from build123d import *

# Parameters (mm, degrees)
BOSS_EXTRUDE1_DEPTH   = 8
FILLET1_R             = 5
FILLET3_R             = 0.5
M4_TAPPED_HOLE1_D     = 3.3
M4_TAPPED_HOLE1_DEPTH = 14.6
M4_TAPPED_HOLE1_TIP   = 0.991420021
M4_TAPPED_HOLE2_D     = 3.3
M4_TAPPED_HOLE2_DEPTH = 14.6
M4_TAPPED_HOLE2_TIP   = 0.991420021


with BuildPart() as part:
    # Sketch1 → Boss-Extrude1 (new body)
    with BuildSketch(Plane.XY):
        Polygon((0, 0), (80, 0), (80, 10), (12, 50), (0, 50), align=None)
    extrude(amount=BOSS_EXTRUDE1_DEPTH)

    # Fillet1
    fillet1_edges = [part.edges().sort_by_distance(p)[0] for p in [
        (12, 50, 4),
        (80, 10, 4),
    ]]
    fillet(fillet1_edges, radius=FILLET1_R)

    # Fillet3
    fillet3_edges = [part.edges().sort_by_distance(p)[0] for p in [
        (0, 50, 4),
        (80, 0, 4),
        (0, 0, 4),
    ]]
    fillet(fillet3_edges, radius=FILLET3_R)

    # M4 Tapped Hole1
    with Locations(Plane.ZY):
        with Locations((4, 43.5), (4, 6)):
            Hole(M4_TAPPED_HOLE1_D / 2, depth=M4_TAPPED_HOLE1_DEPTH)
            with Locations((0, 0, -(M4_TAPPED_HOLE1_DEPTH + M4_TAPPED_HOLE1_TIP / 2))):  # 118° drill point
                Cone(0, M4_TAPPED_HOLE1_D / 2, M4_TAPPED_HOLE1_TIP, mode=Mode.SUBTRACT)

    # M4 Tapped Hole2
    with Locations(Plane(origin=(0, 0, 0), x_dir=(-1, 0, 0), z_dir=(0, -1, 0))):
        with Locations((-20, -4), (-65, -4)):
            Hole(M4_TAPPED_HOLE2_D / 2, depth=M4_TAPPED_HOLE2_DEPTH)
            with Locations((0, 0, -(M4_TAPPED_HOLE2_DEPTH + M4_TAPPED_HOLE2_TIP / 2))):  # 118° drill point
                Cone(0, M4_TAPPED_HOLE2_D / 2, M4_TAPPED_HOLE2_TIP, mode=Mode.SUBTRACT)


solid = part.part
Read the model definition and answer for the solid it produces. Units are mm, in the model's axes. A direction names the side the tool comes from. Round coordinates to 2 decimals unless told otherwise and drop trailing zeros. Order: outer loops, then holes, each group sorted by start corner. A loop starts at its lowest first (then second) coordinate and runs counter-clockwise, first axis right, second up. Notation, with made-up numbers: (42, 83.5) - (51, 83.5) arc R10 ccw to (51, 90.5) - close; hole circle Ø2 at (7.25, 71.25). An arc over 180 degrees is marked (long way). Use one line per item in the form item = value. Start each with the question number.
(1) For faces 1 (the face through (63.35, 7.4, 3.93)), 2 (the face through (11.97, 49.82, 4.06)), 3 (the face through (7.4, 5, 5.31)), determine the directions among +Z, -Z, +X, -X, +Y, -Y from which every point of the face is accessible in a straight line to the end or side of a thin tool.
(2) Find the intervals of material crossed by line 1 along Z through (x, y) = (20, 7); line 2 along Y through (x, z) = (15, 4.25); line 3 along X through (y, z) = (10.5, 4), in increasing order. Write a range as from..to.
(3) The part is cut by section D-D (x = 75). Give the vertices of the cut face in (y, z), then the cut area to 3 significant figures.
(4) Determine the mould class of faces 4 (the face through (31, 20, 8)), 5 (the face through (80, 4, 4)), 6 (the face through (18.69, 7.4, 5)), 7 (the face through (64.7, 15.4, 3.9)) for opening direction X: +X half, -X half, draft (parallel to the pull), parting line (faces both ways), or undercut.
(5) Flat-ended cylindrical pins translate along their axes: pin 1 Ø4 at (y, z) = (30.5, 2) entering from +X; pin 2 Ø3 at (x, z) = (65, 4) entering from +Y; pin 3 Ø2 at (y, z) = (43.5, 4) entering from +X. Find the tip coordinate at first contact, or state that the pin passes through.
(6) The part is cut by section B-B (z = 7). Give the vertices of the cut face in (x, y), then the cut area to 3 significant figures.
(7) The part is cut by section C-C (y = 30). Give the vertices of the cut face in (x, z).
(8) The part is cut by section A-A (y = 12.5). Give the vertices of the cut face in (x, z).
Checked values:
q1.face_1 = -Y
q1.face_2 = +Z, -Z, +X, +Y
q1.face_3 = -X
q2.line_1 = 0..2.35, 5.65..8
q2.line_2 = 0..5.05, 6.95..42.55, 44.45..48.24
q2.line_3 = 0..18.35, 21.65..63.35, 66.65..78.7
q3.outline = (0, 0) - (12.94, 0) - (12.94, 8) - (0, 8) - close
q3.area = 104 mm^2
q4.face_4 = draft
q4.face_5 = +X half
q4.face_6 = undercut
q4.face_7 = undercut
q5.pin_1 = 48.55
q5.pin_2 = 19.71
q5.pin_3 = 24.75
q6.outline = (0, 0.5) arc R0.5 ccw to (0.5, 0) - (79.5, 0) arc R0.5 ccw to (80, 0.5) - (80, 7.14) arc R5 ccw to (77.54, 11.45) - (13.17, 49.31) arc R5 ccw to (10.64, 50) - (0.5, 50) arc R0.5 ccw to (0, 49.5) - close
q6.area = 2,640 mm^2
q7.outline = (0, 0) - (46, 0) - (46, 8) - (0, 8) - close
q8.outline = (0, 0) - (75.75, 0) - (75.75, 8) - (0, 8) - close; hole circle Ø3.3 at (20, 4); hole circle Ø3.3 at (65, 4)
